Can you work these out from the drawing? Everything is in mm from the part's minimum corner. Coordinates: 2 decimals unless noted, no trailing zeros. Order: outer loops, then holes, each group sorted by start corner. A loop starts at its lowest first (then second) coordinate and runs counter-clockwise, first axis right, second up. Notation, with made-up numbers: (7, 44) -> (49, 44) arc R20 ccw to (49, 61) -> close; hole circle Ø9 at (-37.75, -6). An arc over 180 degrees is marked (long way). Use a Markdown table: item, result. Add a question column.
1) If we section it at D-D (z = 38): Write out the boundary of the cut face in (x, y).
2) If we section it at A-A (z = 47.5): Write out the boundary of the cut face in (x, y), plus the area to 3 significant figures.
3) If I drill on L1, parallel to X at y = 6.75, z = 47.5; L2, parallel to Z at x = 59.5, y = 8; L3, parallel to Z at x = 44.5, y = 4, over which ranges is the centre line in solid material (lowest first)? Write a range as [from, to].
4) Will these pins go through, and if not, where does the flat tip stop? pin 1 Ø3.5 at (x, z) = (47.5, 6.25) entering from +Y; pin 2 Ø2 at (x, y) = (21, 3) entering from +Z; pin 3 Ø2 at (y, z) = (6, 16) entering from -X; pin 4 Ø1.5 at (x, y) = (35, 5) entering from -Z.
5) If we section it at B-B (x = 47.5): Write out the boundary of the cut face in (y, z).
6) Thinking about a two-plate mould opening in X: for the marked faces 1, 2 and 3, which applies, +X half, -X half, draft (parallel to the pull), parting line (faces both ways), or undercut?
7) If we section it at C-C (y = 4.25): Write out the boundary of the cut face in (x, z).
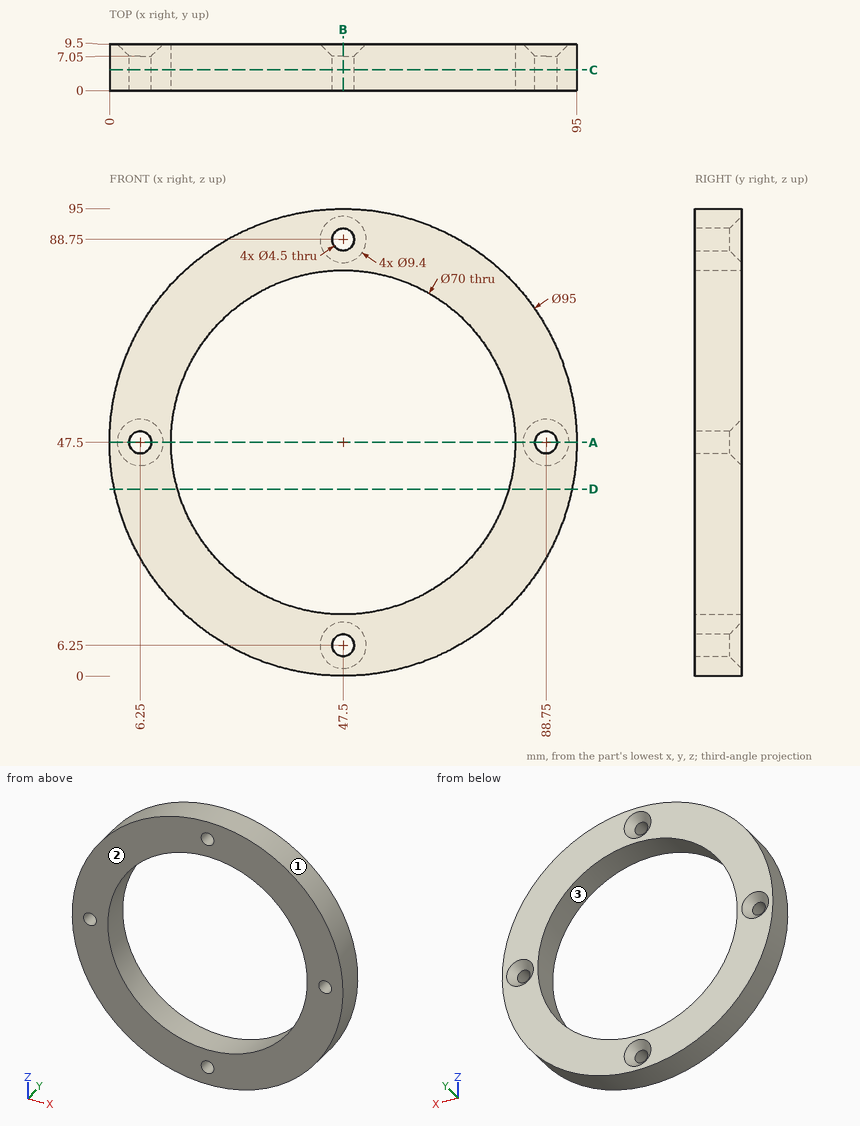
Answer sheet:
| question | item | result |
|---|---|---|
| 1 | outline | (0.96, 0) -> (13.81, 0) -> (13.81, 9.5) -> (0.96, 9.5) -> close; (81.19, 0) -> (94.04, 0) -> (94.04, 9.5) -> (81.19, 9.5) -> close |
| 2 | outline | (0, 0) -> (4, 0) -> (4, 7.05) -> (1.55, 9.5) -> (0, 9.5) -> close; (8.5, 0) -> (12.5, 0) -> (12.5, 9.5) -> (10.95, 9.5) -> (8.5, 7.05) -> close; (82.5, 0) -> (86.5, 0) -> (86.5, 7.05) -> (84.05, 9.5) -> (82.5, 9.5) -> close; (91, 0) -> (95, 0) -> (95, 9.5) -> (93.45, 9.5) -> (91, 7.05) -> close |
| 2 | area | 140 mm2 |
| 3 | L1 | [0, 4], [8.5, 12.5], [82.5, 86.5], [91, 95] |
| 3 | L2 | [1.54, 14.62], [80.38, 93.46] |
| 3 | L3 | [0.09, 12.63], [82.37, 94.91] |
| 4 | pin 1 | through |
| 4 | pin 2 | z = 87.57 |
| 4 | pin 3 | x = 11.09 |
| 4 | pin 4 | z = 1.48 |
| 5 | outline | (0, 0) -> (9.5, 0) -> (9.5, 1.55) -> (7.05, 4) -> (0, 4) -> close; (0, 8.5) -> (7.05, 8.5) -> (9.5, 10.95) -> (9.5, 12.5) -> (0, 12.5) -> close; (0, 82.5) -> (9.5, 82.5) -> (9.5, 84.05) -> (7.05, 86.5) -> (0, 86.5) -> close; (0, 91) -> (7.05, 91) -> (9.5, 93.45) -> (9.5, 95) -> (0, 95) -> close |
| 6 | face 1 | parting line |
| 6 | face 2 | draft |
| 6 | face 3 | undercut |
| 7 | outline | circle Ø95 at (47.5, 47.5); hole circle Ø4.5 at (6.25, 47.5); hole circle Ø70 at (47.5, 47.5); hole circle Ø4.5 at (47.5, 6.25); hole circle Ø4.5 at (47.5, 88.75); hole circle Ø4.5 at (88.75, 47.5) |
